Input: part model. Units: mm. Frame: model coordinates. Face numbers are marked on the shaded views. A direction names the side the tool comes from. Coordinates: 2 decimals unless noted, no trailing zeros. Loops run counter-clockwise (first coordinate to the right, second up) from the corner with the lowest first, then second, coordinate; pieces in that order, holes last. Notation, with made-up numbers: (-15, 18.5) - (-8, 18.5) arc R7 ccw to (-8, 27.5) - close; hole circle Ø3 at (-14.75, -25). An arc over 180 degrees is marked (long way). Use a Markdown table: item, result. Add a question column.
1. Access query for the marked faces 4 and 5. Directions: +Z, -Z, +X, -X, +Y, -Y. A direction counts if a zero-diameter tool reaches every point of the face in a straight line with its end or side. Return the directions, or none.
2. Section query A-A on z = 5. Return the cut outline in (x, y).
3. Draft query along Y for the marked faces 1, 2 and 3. Return one class per face: released by +Y, released by -Y, zero draft, split by the parting line, or undercut.
4. Section query C-C on z = 13.5. Return the cut outline in (x, y), then the cut area to 3 significant figures.
5. Ray query, L1, parallel to Y at x = 0, z = 5.75; L2, parallel to X at y = 0, z = 7.25; L3, parallel to X at y = 0, z = 14.75. Return the intervals inside material, ascending. Write a range as [from, to].
6. Contact query for flat-ended pins moving along their axis: P1, Ø1, axis at y = -4.5, z = 9.5, coming from the +X side; P2, Ø1.5, axis at x = -4, z = 18, coming from the +Y side; P3, Ø2, axis at y = 1.5, z = 11, coming from the +X side. Output: stop coordinate, or through.
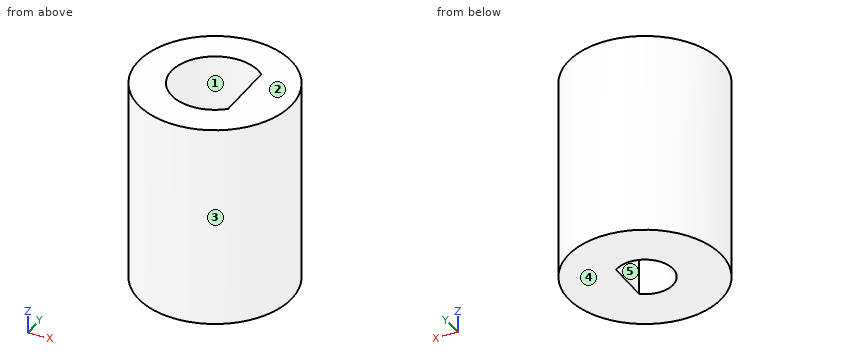
Autodesk Fusion 360 part; units mm, degrees
sketch "Sketch5" plane through (0, 0, 0) normal (0, 0, 1) x (1, 0, 0)
  circle A0 centre (0, 0) radius 7.5
  line L0 (1.7, 2.1616) -> (1.7, -2.1616)
  arc A1 (1.7, 2.1616) -> (1.7, -2.1616) centre (0, 0) ccw
  dimension "d19" = 15
  dimension "d29" = 5.5
  dimension "d30" = 1.7
extrude "Extrude7" add sketch "Sketch5" along normal blind 10
sketch "Sketch7" plane through (0, 0, 10) normal (0, 0, 1) x (-1, 0, 0)
  arc A0 (-1.7, -2.1616) -> (-1.7, 2.1616) centre (0, 0) ccw
  line L0 (-1.7, -2.1616) -> (-1.7, 2.1616)
  circle A1 centre (0, 0) radius 7.5
  circle A2 centre (0, 0) radius 7.5
  line L1 (-2.9, -3.1068) -> (-2.9, 3.1068)
  arc A3 (-2.9, -3.1068) -> (-2.9, 3.1068) centre (0, 0) ccw
  dimension "d35" = 8.5
  dimension "d36" = 2.9
extrude "Extrude8" add sketch "Sketch7" along normal blind 10 contours A1 A2
Resolved:
| question | item | result |
|---|---|---|
| 1 | face 4 | -Z, +X, -X, +Y, -Y |
| 1 | face 5 | +Z, -Z |
| 2 | outline | circle Ø15 at (0, 0); hole (1.7, -2.16) - (1.7, 2.16) arc R2.75 ccw (long way) to start |
| 3 | face 1 | undercut |
| 3 | face 2 | zero draft |
| 3 | face 3 | split by the parting line |
| 4 | outline | circle Ø15 at (0, 0); hole (2.9, -3.11) - (2.9, 3.11) arc R4.25 ccw (long way) to start |
| 4 | area | 126 mm² |
| 5 | L1 | [-7.5, -2.75], [2.75, 7.5] |
| 5 | L2 | [-7.5, -2.75], [1.7, 7.5] |
| 5 | L3 | [-7.5, -4.25], [2.9, 7.5] |
| 6 | P1 | x = 6.34 |
| 6 | P2 | y = 6.76 |
| 6 | P3 | x = 7.48 |
